For this review, take the finished solid that the model builds, in its own axes (mm). Coordinates: 2 decimals unless noted, no trailing zeros. Loops run counter-clockwise (first coordinate to the right, second up) from the corner with the lowest first, then second, coordinate; pieces in that order, holes last. Notation, with made-up numbers: (-23, 33) -> (15, 33) arc R7 ccw to (15, 42) -> close; hole circle Ø2 at (1.5, -40). An arc over 180 degrees is marked (long way). Answer in a Markdown table with one row per item.
from build123d import *

# Parameters (mm, degrees)
SKETCH_1_R      = 8.5
SKETCH_1_R_2    = 1.6
EXTRUDE_1_DEPTH = 1
FILLET_1_R      = 10


with BuildPart() as part:
    # Эскиз1 → Бобышка-Вытянуть1 (new body)
    with BuildSketch(Plane(origin=(0, 0, 0), x_dir=(0, 0, -1), z_dir=(1, 0, 0))):
        with BuildLine():
            ThreePointArc((11.473333333, -6.404859266), (23.78, 0), (11.473333333, 6.404859266))
            ThreePointArc((11.473333333, 6.404859266), (-13.14, 0), (11.473333333, -6.404859266))
        make_face()
        Circle(SKETCH_1_R, mode=Mode.SUBTRACT)
        with Locations((15.96, 0)):
            Circle(SKETCH_1_R_2, mode=Mode.SUBTRACT)
    extrude(amount=EXTRUDE_1_DEPTH)

    # Скругление1
    fillet_1_edges = [part.edges().sort_by_distance(p)[0] for p in [
        (0.5, -6.404859266, -11.473333333),
        (0.5, 6.404859266, -11.473333333),
    ]]
    fillet(fillet_1_edges, radius=FILLET_1_R)


solid = part.part
Item 1: The part is to be moulded in two halves that separate along Z. For faces 1 (the cylindrical face through (0.493, 0.417, 13.133)), 2 (the cylindrical face through (0.493, 0.481, -17.486)), 3 (the flat face through (0, 0, -9)), say which applies: +Z half, -Z half, draft (parallel to the pull), parting line (faces both ways), or undercut.
Worked answers:
| item | result |
|---|---|
| face 1 | parting line |
| face 2 | undercut |
| face 3 | draft |
Item 2: Take a section at B-B, the plane y = 0. State the section outline as (x, z) points.
Worked answers:
| item | result |
|---|---|
| outline | (0, -23.78) -> (1, -23.78) -> (1, -17.56) -> (0, -17.56) -> close; (0, -14.36) -> (1, -14.36) -> (1, -8.5) -> (0, -8.5) -> close; (0, 8.5) -> (1, 8.5) -> (1, 13.14) -> (0, 13.14) -> close |
Item 3: Take a section at D-D, the plane x = 0.6. Count the separate pieces of the cut face and the enclosed holes in it, and give its area (3 significant figures).
Worked answers:
| item | result |
|---|---|
| separate pieces | 1 |
| enclosed holes | 2 |
| area | 464 mm² |
Item 4: Take a section at A-A, the plane z = 0. State the section outline as (x, y) points.
Worked answers:
| item | result |
|---|---|
| outline | (0, -13.14) -> (1, -13.14) -> (1, -8.5) -> (0, -8.5) -> close; (0, 8.5) -> (1, 8.5) -> (1, 13.14) -> (0, 13.14) -> close |
Item 5: Take a section at C-C, the plane z = -15.96. State the section outline as (x, y) points.
Worked answers:
| item | result |
|---|---|
| outline | (0, -7.82) -> (1, -7.82) -> (1, -1.6) -> (0, -1.6) -> close; (0, 1.6) -> (1, 1.6) -> (1, 7.82) -> (0, 7.82) -> close |
Item 6: For L1, parallel to Y at x = 0.5, z = 0; L2, parallel to Y at x = 0.15, z = -16; L3, parallel to Z at x = 0.5, y = 6.5, list the stretches that pass through material, from the lowest coordinate up.
Worked answers:
| item | result |
|---|---|
| L1 | -13.14 to -8.5, 8.5 to 13.14 |
| L2 | -7.82 to -1.6, 1.6 to 7.82 |
| L3 | -20.31 to -5.48, 5.48 to 11.42 |
